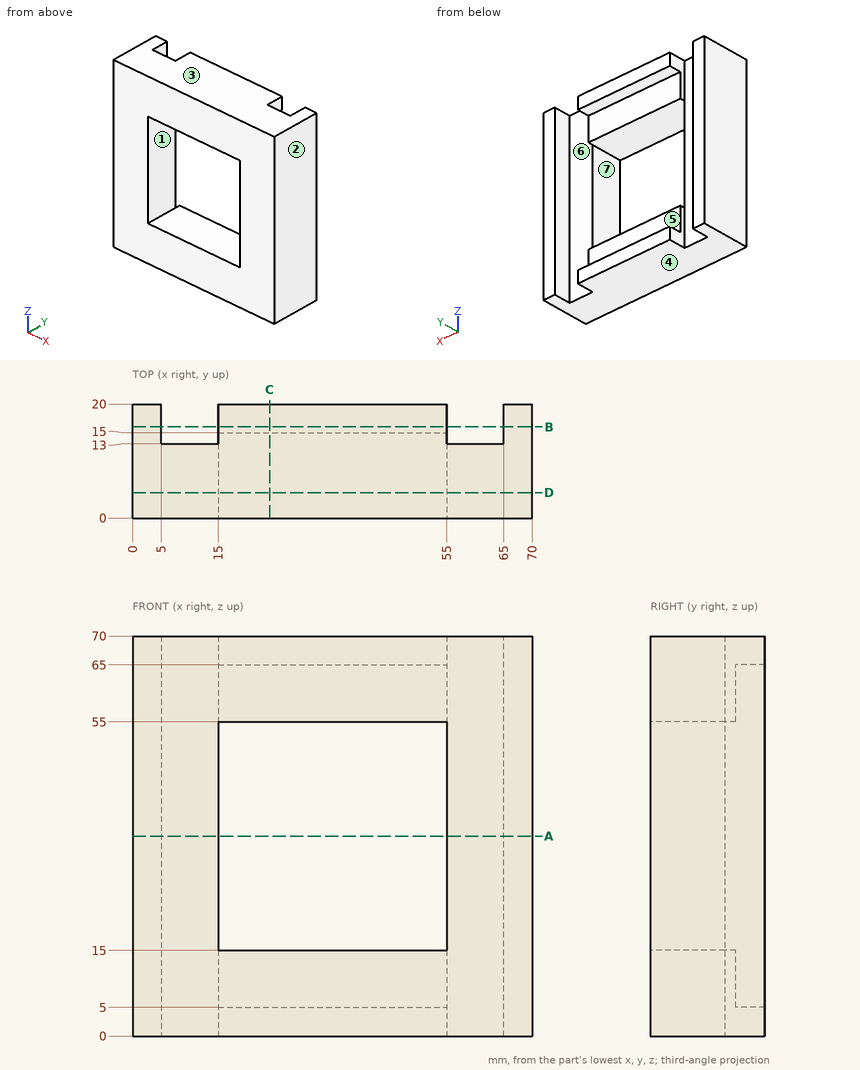
Answer from the drawing. Dimensions are ordinates in mm from the lowest x, y and z of the part. A direction names the side the tool comes from. Give positions to 0.01 mm unless a question says otherwise; leave off trailing zeros. Write each loop counter-clockwise with the first axis right and the second up, starting at its lowest first coordinate (ties: lowest second). Pieces come first, ordered by that corner, then holes.
1) Section C-C (x = 24) is taken. Write down the section's boundary in (y, z), and give its area (3 significant figures).
2) Section A-A (z = 35) is taken. Write down the section's boundary in (x, y).
3) Section B-B (y = 16) is taken. Write down the section's boundary in (x, z).
4) Section D-D (y = 4.5) is taken. Write down the section's boundary in (x, z).
5) Given P1, Ø1, axis at x = 18.5, z = 57, coming from the -Y side; P2, Ø3, axis at x = 8.5, z = 19, coming from the +Y side; P3, Ø11, axis at x = 36, z = 12.5, coming from the +Y side; P4, Ø10, axis at x = 24, z = 26, coming from the -Y side, each flat-ended and moving along its own axis, determine where each tip first touches the part or whether it passes through.
6) Find the intervals of material crossed by L1, parallel to Z at x = 47, y = 18.75; L2, parallel to Z at x = 41.5, y = 9, in increasing order.
7) A tool of negligible diameter and unlimited length cuts with its end or side. For the marked faces 4, 5, 6 and 7, from which of +Z, -Z, +X, -X, +Y, -Y can it reach the whole face along a straight path? Write none if from no direction.
8) For a pull along X with two mould halves and no side action, classify the marked faces 1, 2 and 3 as pulls with the +X half, pulls with the -X half, needs draft (parallel to the pull), parting line crosses it, or undercut.
Response:
1. outline: (0, 0) - (20, 0) - (20, 5) - (15, 5) - (15, 15) - (0, 15) - close; (0, 55) - (15, 55) - (15, 65) - (20, 65) - (20, 70) - (0, 70) - close
1. area: 500 mm2
2. outline: (0, 0) - (15, 0) - (15, 13) - (5, 13) - (5, 20) - (0, 20) - close; (55, 0) - (70, 0) - (70, 20) - (65, 20) - (65, 13) - (55, 13) - close
3. outline: (0, 0) - (5, 0) - (5, 70) - (0, 70) - close; (15, 0) - (55, 0) - (55, 5) - (15, 5) - close; (15, 65) - (55, 65) - (55, 70) - (15, 70) - close; (65, 0) - (70, 0) - (70, 70) - (65, 70) - close
4. outline: (0, 0) - (70, 0) - (70, 70) - (0, 70) - close; hole (15, 15) - (55, 15) - (55, 55) - (15, 55) - close
5. P1: stops at y = 0
5. P2: stops at y = 13
5. P3: stops at y = 15
5. P4: passes through
6. L1: z = 0 to 5, 65 to 70
6. L2: z = 0 to 15, 55 to 70
7. face 4: -Z, +X, -X, +Y, -Y
7. face 5: +Y
7. face 6: +Z, -Z, +Y
7. face 7: +Y, -Y
8. face 1: undercut
8. face 2: pulls with the +X half
8. face 3: needs draft
